Job drawing, mm, ordinate dimensions from the low corner. One solid piece. A direction names the side the tool comes from. Round coordinates to 2 decimals unless told otherwise and drop trailing zeros. Write each loop counter-clockwise with the first axis right and the second up, starting at its lowest first coordinate (ties: lowest second). Pieces come first, ordered by that corner, then holes. Notation, with made-up numbers: M 52,85 L 59,85 A12 ccw 59,89 Z; hole C 41,50.5 d1. An arc over 180 degrees is marked long. Answer as a JSON object with one key per item and string values. Group by question number.
1. Band-saw the part on C-C, the plane y = 5.5. Write the cut outline in (x, z).
2. Two-plate mould, pull along Y, no slides. Class the marked faces 1, 2 and 3: +Y half, -Y half, draft (parallel to the pull), parting line (faces both ways), or undercut.
3. Drop flat-ended pins along their axis: pin 1 (2.5 mm diameter, centred on x = 31, z = 4, fed in from +Y); pin 2 (2.5 mm diameter, centred on x = 30, z = 5.5, fed in from -Y); pin 3 (3 mm diameter, centred on y = 26, z = 2.5, fed in from +X). Give the stop position or say it passes through.
4. Which spindle directions (+Z, -Z, +X, -X, +Y, -Y) get a long thin tool onto all of the face, cutting with end or side? Do the marked faces 4, 5, 6, 7 and 8. Say none if no direction does.
5. Band-saw the part on A-A, the plane x = 31.5. Write the cut outline in (y, z).
6. Drill centre lines: line 1 (Y direction, x = 28.5, z = 3); line 2 (Y direction, x = 27.5, z = 11.25); line 3 (X direction, y = 23, z = 7.25). Where is each one in solid material? Low to high. Write a range as from..to.
7. Band-saw the part on D-D, the plane x = 6.5. Write the cut outline in (y, z).
8. Band-saw the part on B-B, the plane z = 2. Write the cut outline in (x, y).
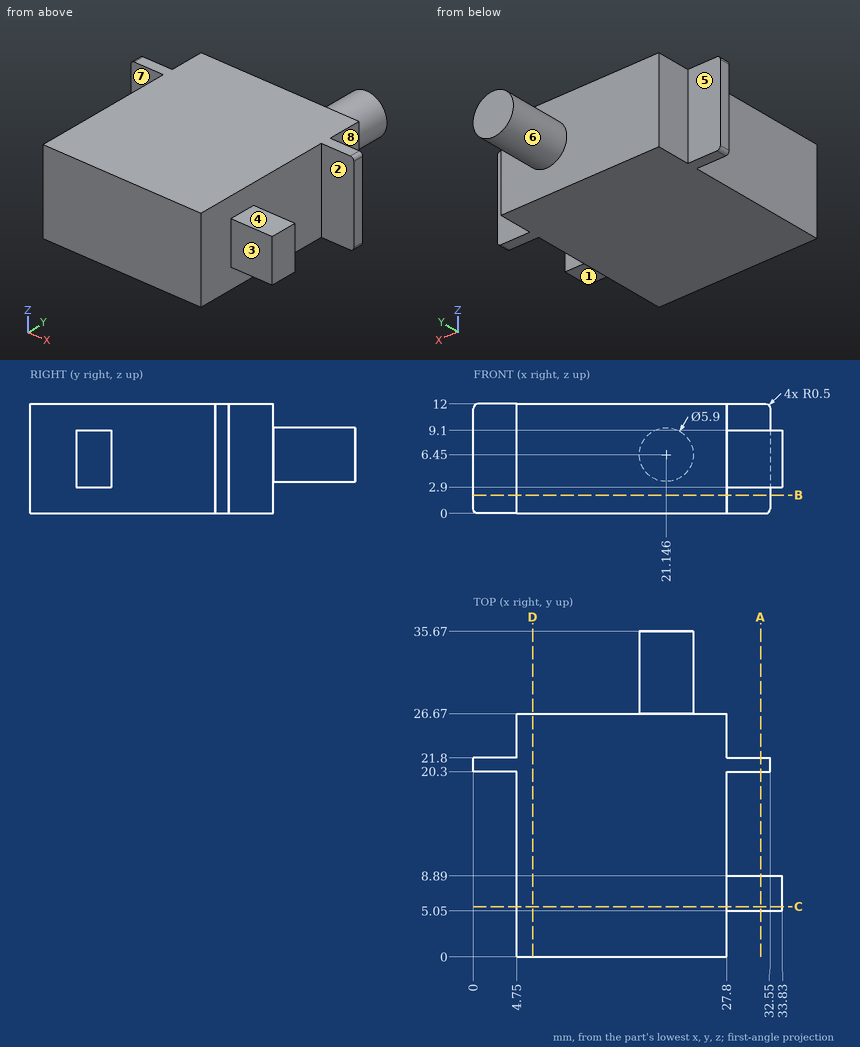
Worked answers:
{
 "1": {"outline": "M 4.75,0 L 27.8,0 L 27.8,2.9 L 33.83,2.9 L 33.83,9.1 L 27.8,9.1 L 27.8,12 L 4.75,12 Z"},
 "2": {"face 1": "draft", "face 2": "undercut", "face 3": "-Y half"},
 "3": {"pin 1": "stops at y = 21.8", "pin 2": "stops at y = 5.05", "pin 3": "stops at x = 27.8"},
 "4": {"face 4": "+Z, +X, -Y", "face 5": "+Z, -Z, -X, +Y", "face 6": "+Y", "face 7": "+Z, -Z, -X, -Y", "face 8": "+Z, -Z, +X, +Y"},
 "5": {"outline": "M 5.05,2.9 L 8.89,2.9 L 8.89,9.1 L 5.05,9.1 Z; M 20.3,0 L 21.8,0 L 21.8,12 L 20.3,12 Z"},
 "6": {"line 1": "y = 5.05..8.89, 20.3..21.8", "line 2": "y = 0..26.67", "line 3": "x = 4.75..27.8"},
 "7": {"outline": "M 0,0 L 26.67,0 L 26.67,12 L 0,12 Z"},
 "8": {"outline": "M 0,20.3 L 4.75,20.3 L 4.75,0 L 27.8,0 L 27.8,20.3 L 32.55,20.3 L 32.55,21.8 L 27.8,21.8 L 27.8,26.67 L 4.75,26.67 L 4.75,21.8 L 0,21.8 Z"}
}
